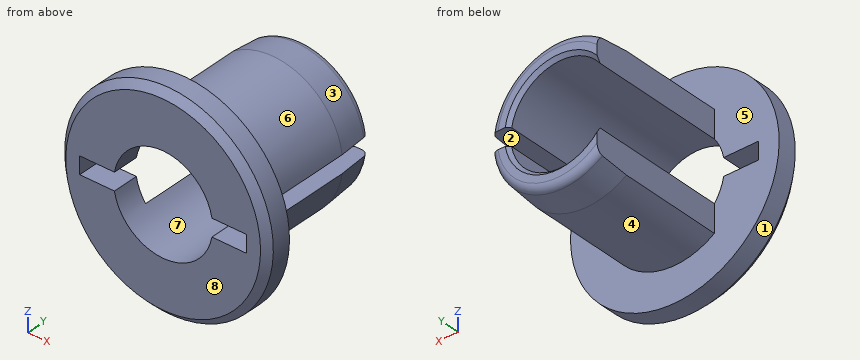
```python
from build123d import *

# Parameters (mm, degrees)
SKETCH2_R             = 3
BOSS_EXTRUDE2_DEPTH   = 0.75
BOSS_EXTRUDE3_DEPTH   = 4
CROQUIS1_R            = 1.425
CORTAR_EXTRUIR1_DEPTH = 7.368869601
CHAFL_N1_SIZE         = 0.2
CHAFL_N2_SIZE         = 1
CHAFL_N2_SIZE2        = 0.087488664
CHAFL_N3_SIZE         = 0.1
REDONDEO1_R           = 0.2
CROQUIS2_W            = 1.845726181
CROQUIS2_H            = 0.5
CORTAR_EXTRUIR2_DEPTH = 7.368869676


with BuildPart() as part:
    # Sketch2 → Boss-Extrude2 (new body)
    with BuildSketch(Plane(origin=(0, 0, 0), x_dir=(-1, 0, 0), z_dir=(0, 1, 0))):
        with Locations(Location((0, 0, 0), (0, 0, 90))):
            Circle(SKETCH2_R)
    extrude(amount=BOSS_EXTRUDE2_DEPTH)

    # Sketch3 → Boss-Extrude3 (add)
    with BuildSketch(Plane(origin=(0, 0.75, 0), x_dir=(-1, 0, 0), z_dir=(0, 1, 0))):
        with BuildLine():
            Line((1.13862177, 1.644244649), (1.13862177, -1.644244649))
            ThreePointArc((1.13862177, -1.644244649), (-2, 0), (1.13862177, 1.644244649))
        make_face()
    extrude(amount=BOSS_EXTRUDE3_DEPTH)

    # Croquis1 → Cortar-Extruir1 (cut, through all)
    with BuildSketch(Plane(origin=(0, 4.75, 0), x_dir=(1, 0, 0), z_dir=(0, 1, 0))):
        with Locations(Location((0, 0, 0), (0, 0, 270))):
            Circle(CROQUIS1_R)
    extrude(amount=-CORTAR_EXTRUIR1_DEPTH, mode=Mode.SUBTRACT)

    # Chaflán1
    chafl_n1_edges = [part.edges().sort_by_distance(p)[0] for p in [
        (0, 0, -3),
    ]]
    chamfer(chafl_n1_edges, length=CHAFL_N1_SIZE)

    # Chaflán2
    chafl_n2_edges = [part.edges().sort_by_distance(p)[0] for p in [
        (2, 4.75, 0),
    ]]
    chafl_n2_side = [part.faces().sort_by_distance(p)[0] for p in [
        (2, 2.75, 0),
    ]]
    chamfer(chafl_n2_edges, length=CHAFL_N2_SIZE, length2=CHAFL_N2_SIZE2, reference=chafl_n2_side[0])

    # Chaflán3
    chafl_n3_edges = [part.edges().sort_by_distance(p)[0] for p in [
        (1.275071419, 4.75, -0.636252996),
    ]]
    chamfer(chafl_n3_edges, length=CHAFL_N3_SIZE)

    # Redondeo1
    redondeo1_edges = [part.edges().sort_by_distance(p)[0] for p in [
        (1.912511336, 4.75, 0),
    ]]
    fillet(redondeo1_edges, radius=REDONDEO1_R)

    # Croquis2 → Cortar-Extruir2 (cut, through all)
    with BuildSketch(Plane.XZ):
        with Locations((1.47713691, 0)):
            Rectangle(CROQUIS2_W, CROQUIS2_H)
    cortar_extruir2 = extrude(amount=-CORTAR_EXTRUIR2_DEPTH, mode=Mode.SUBTRACT)

    # Simetría1: Cortar-Extruir2 across plane
    add(cortar_extruir2.mirror(Plane(origin=(0, 0, 0), x_dir=(0, 0, 1), z_dir=(1, 0, 0))), mode=Mode.SUBTRACT)


solid = part.part
```
Input: part model. Units: mm. Frame: model coordinates. Face numbers are marked on the shaded views. A direction names the side the tool comes from. Give positions to 0.01 mm unless a question says otherwise; leave off trailing zeros. Order: outer loops, then holes, each group sorted by start corner. A loop starts at its lowest first (then second) coordinate and runs counter-clockwise, first axis right, second up. Notation, with made-up numbers: M 28.25,85.5 L 62.25,85.5 A25 cw 62.25,99.5 Z; hole C -25.75,28.25 d6. An arc over 180 degrees is marked long. One line per question, with ' | ' between items. Start each with the question number.
1. Section query C-C (y = 4.45). Return the cut outline in (x, z) (3 decimals), and give its area (3 significant figures).
2. Pull-direction query (Z, two-part tool) for the marked faces 1, 2 and 3; classes: released by +Z, released by -Z, zero draft, split by the parting line, or undercut.
3. First-contact query: pin 1 Ø3 at (x, z) = (0.5, 1) entering from +Y; pin 2 Ø0.8 at (x, y) = (2, 2.5) entering from +Z; pin 3 Ø1 at (y, z) = (1, 1) entering from -X; pin 4 Ø2 at (y, z) = (3.5, 1.5) entering from -X. Flat tips, straight axial feed; report the tip coordinate or a pass-through.
4. Section query A-A (z = 0). Return the cut outline in (x, y), and give its area (3 significant figures).
5. Section query B-B (y = 3.65). Return the cut outline in (x, z) (3 decimals), and give its area (3 significant figures).
6. Material intervals for probe 1 along Y at (x, z) = (-2.2, 1.05); probe 2 along Z at (x, y) = (-1.9, 0.7); probe 3 along X at (y, z) = (3.65, -1.25), sorted ascending. Write a range as [from, to].
7. Access query for the marked faces 4, 5, 6, 7 and 8. Directions: +Z, -Z, +X, -X, +Y, -Y. A direction counts if a zero-diameter tool reaches every point of the face in a straight line with its end or side. Return the directions, or none.
Here are the results:
1) outline: M -1.139,-1.569 A1.939 ccw 1.923,-0.25 L 1.403,-0.25 A1.425 cw -1.139,-0.857 Z; M -1.139,0.857 A1.425 cw 1.403,0.25 L 1.923,0.25 A1.939 ccw -1.139,1.569 Z | area: 3.75 mm²
2) face 1: split by the parting line | face 2: undercut | face 3: released by +Z
3) pin 1: y = 4.75 | pin 2: z = 1.2 | pin 3: x = -2.95 | pin 4: x = -1.14
4) outline: M -3,0.2 L -2.8,0 L -2.4,0 L -2.4,0.75 L -3,0.75 Z; M 2.4,0 L 2.8,0 L 3,0.2 L 3,0.75 L 2.4,0.75 Z | area: 0.860 mm²
5) outline: M -1.139,-1.644 A2 ccw 1.984,-0.25 L 1.403,-0.25 A1.425 cw -1.139,-0.857 Z; M -1.139,0.857 A1.425 cw 1.403,0.25 L 1.984,0.25 A2 ccw -1.139,1.644 Z | area: 4.24 mm²
6) probe 1: [0, 0.75] | probe 2: [-2.32, -0.25], [0.25, 2.32] | probe 3: [-1.14, -0.68], [0.68, 1.56]
7) face 4: -Z, +Y | face 5: +Y | face 6: +Z, +Y | face 7: +Y, -Y | face 8: +Z, -Z, +X, -X, -Y
